Verification items for this drawing (mm, ordinates from the low corner). A direction names the side the tool comes from. Coordinates: 2 decimals unless noted, no trailing zeros. Write each loop counter-clockwise with the first axis right and the second up, starting at its lowest first coordinate (ties: lowest second). Pieces come first, ordered by that corner, then holes. Notation, with made-up numbers: (-27, 3) -> (3, 3) arc R26 cw to (3, 42) -> close; hole circle Ø5 at (64.5, -11). An arc over 180 degrees is marked (long way). Use CSV: the item, a comma, the result in double quotes.
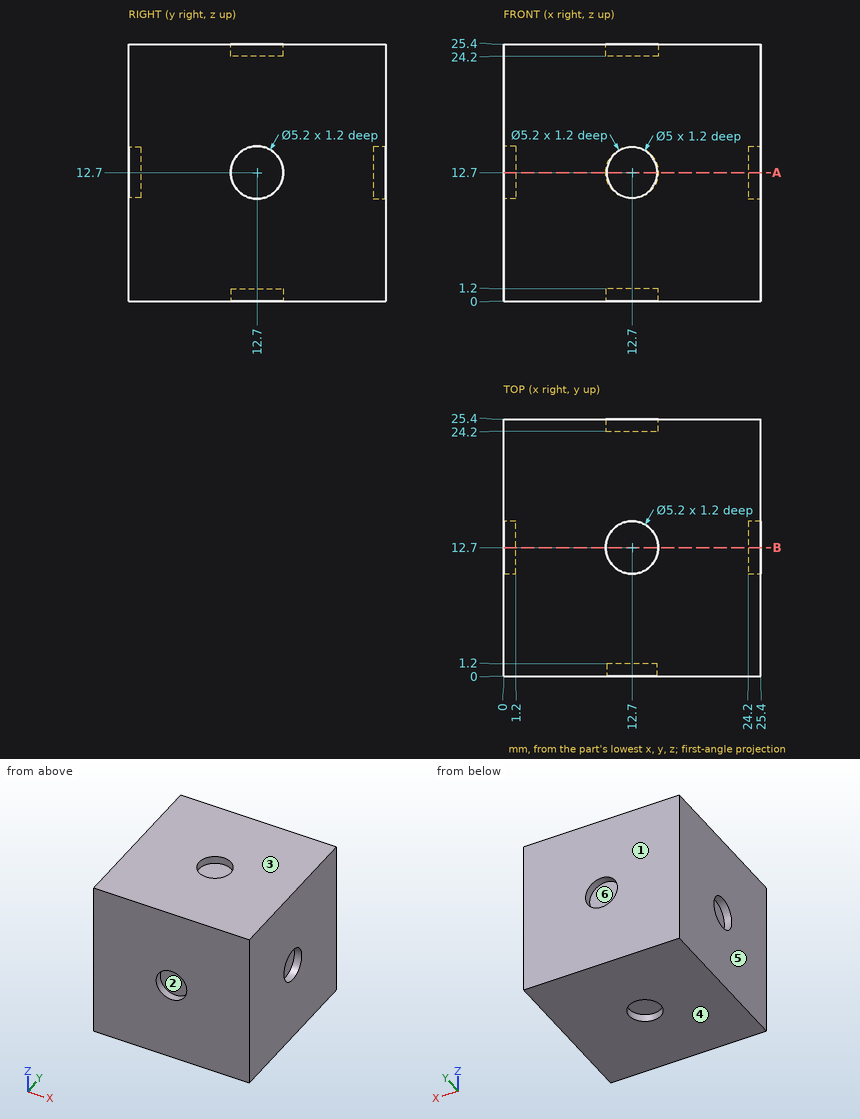
1) Cross-section at B-B (y = 12.7). Record the boundary of the cut face in (x, z).
Return value:
outline,"(0, 0) -> (10.1, 0) -> (10.1, 1.2) -> (15.3, 1.2) -> (15.3, 0) -> (25.4, 0) -> (25.4, 10.1) -> (24.2, 10.1) -> (24.2, 15.3) -> (25.4, 15.3) -> (25.4, 25.4) -> (15.3, 25.4) -> (15.3, 24.2) -> (10.1, 24.2) -> (10.1, 25.4) -> (0, 25.4) -> (0, 15.3) -> (1.2, 15.3) -> (1.2, 10.1) -> (0, 10.1) -> close"
2) Set-up check for the marked faces 5 and 6: record each of +Z, -Z, +X, -X, +Y, -Y from which the full face is reachable in a straight line by a thin tool's end or side.
Return value:
face 5,"+Z, -Z, -X, +Y, -Y"
face 6,"+Y"
3) Gauge pin test, flat ends, axial feed: pin 1 (2.5 mm diameter, centred on x = 12.5, z = 13.5, fed in from -Y); pin 2 (4 mm diameter, centred on x = 12.5, z = 13, fed in from +Y); pin 3 (8 mm diameter, centred on x = 19.5, z = 8.5, fed in from -Y); pin 4 (2.5 mm diameter, centred on x = 13, y = 13, fed in from +Z). Record the tip position at first contact, or that the pin passes through.
Return value:
pin 1,"y = 1.2"
pin 2,"y = 24.2"
pin 3,"y = 0"
pin 4,"z = 24.2"
4) Mould release check, pull along Z, two halves, no side actions. Record for the marked faces 1, 2, 3 and 4: released by +Z, released by -Z, zero draft, split by the parting line, or undercut.
Return value:
face 1,"zero draft"
face 2,"undercut"
face 3,"released by +Z"
face 4,"released by -Z"
5) Cross-section at A-A (z = 12.7). Record the boundary of the cut face in (x, y), plus the area to 3 significant figures.
Return value:
outline,"(0, 0) -> (10.2, 0) -> (10.2, 1.2) -> (15.2, 1.2) -> (15.2, 0) -> (25.4, 0) -> (25.4, 10.1) -> (24.2, 10.1) -> (24.2, 15.3) -> (25.4, 15.3) -> (25.4, 25.4) -> (15.3, 25.4) -> (15.3, 24.2) -> (10.1, 24.2) -> (10.1, 25.4) -> (0, 25.4) -> (0, 15.3) -> (1.2, 15.3) -> (1.2, 10.1) -> (0, 10.1) -> close"
area,"620 mm2"
6) Scan lines: L1, parallel to Z at x = 12.7, y = 0.45; L2, parallel to Z at x = 0.65, y = 12.7. Record each from-to range of solid material in increasing order.
Return value:
L1,"0 to 10.2, 15.2 to 25.4"
L2,"0 to 10.1, 15.3 to 25.4"
